Here's the drawing with two shaded views (mm, measured from the low corner). I have some questions. Give positions to 0.01 mm unless a question says otherwise; leave off trailing zeros. Write each question's results on one line, items separated by ' | '. Start each with the question number.
Q1. If I drill on line 1 along X through (y, z) = (42, 49) (1 decimal); line 2 along X through (y, z) = (12.5, 50) (1 decimal); line 3 along Y through (x, z) = (8.5, 38) (1 decimal), over which ranges is the centre line in solid material (lowest first)?
Q2. If we section it at B-B, the plane y = 50: Give the number of separate pieces and of enclosed holes in the cut face, plus the area to 3 significant figures.
Q3. Will these pins go through, and if not, where does the flat tip stop? P1, Ø3, axis at x = 19.5, z = 28.5, coming from the -Y side; P2, Ø2, axis at x = 18.5, y = 50.5, coming from the -Z side (1 decimal); P3, Ø3, axis at x = 25.5, y = 42, coming from the +Z side.
Q4. We'd pull the mould along X, two halves only. Please class the marked faces 1, 2 and 3: released by +X, released by -X, zero draft, split by the parting line, or undercut.
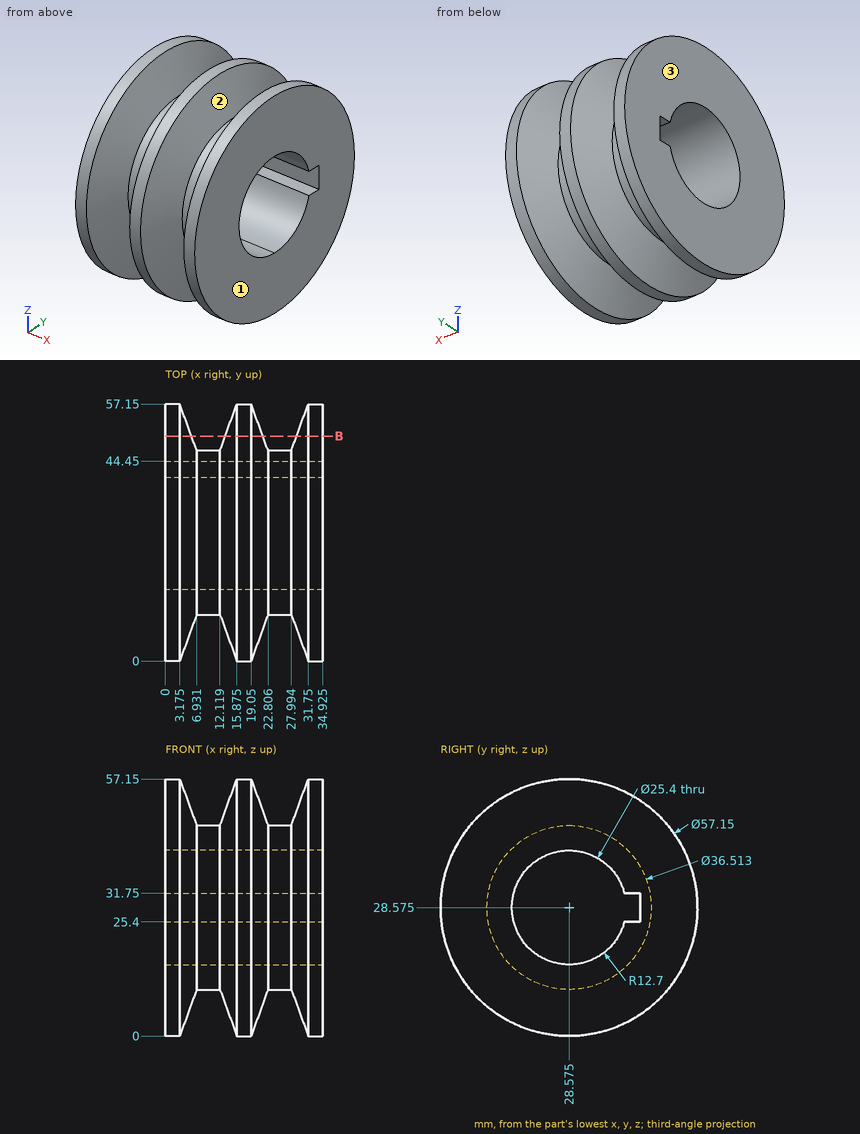
Final values:
1) line 1: x = 0 to 4.7, 14.4 to 20.6, 30.2 to 34.9 | line 2: x = 0 to 3.8, 15.2 to 19.7, 31.1 to 34.9 | line 3: y = 12.9 to 20.1, 37.1 to 44.2
2) separate pieces: 3 | enclosed holes: 0 | area: 615 mm²
3) P1: stops at y = 0 | P2: stops at z = 9.1 | P3: stops at z = 42.4
4) face 1: released by +X | face 2: undercut | face 3: released by -X
